Print and shaded views of the part. All mm, measured from the part's lowest x, y and z. Coordinates: 2 decimals unless noted, no trailing zeros. Write each loop counter-clockwise with the first axis right and the second up, starting at its lowest first coordinate (ties: lowest second). Pieces come first, ordered by that corner, then holes. Notation, with made-up numbers: (-17, 0) -> (6, 0) arc R24 ccw to (6, 36) -> close; hole circle Ø8 at (-4, 77). An arc over 180 degrees is marked (long way). Write item = value, one per line.
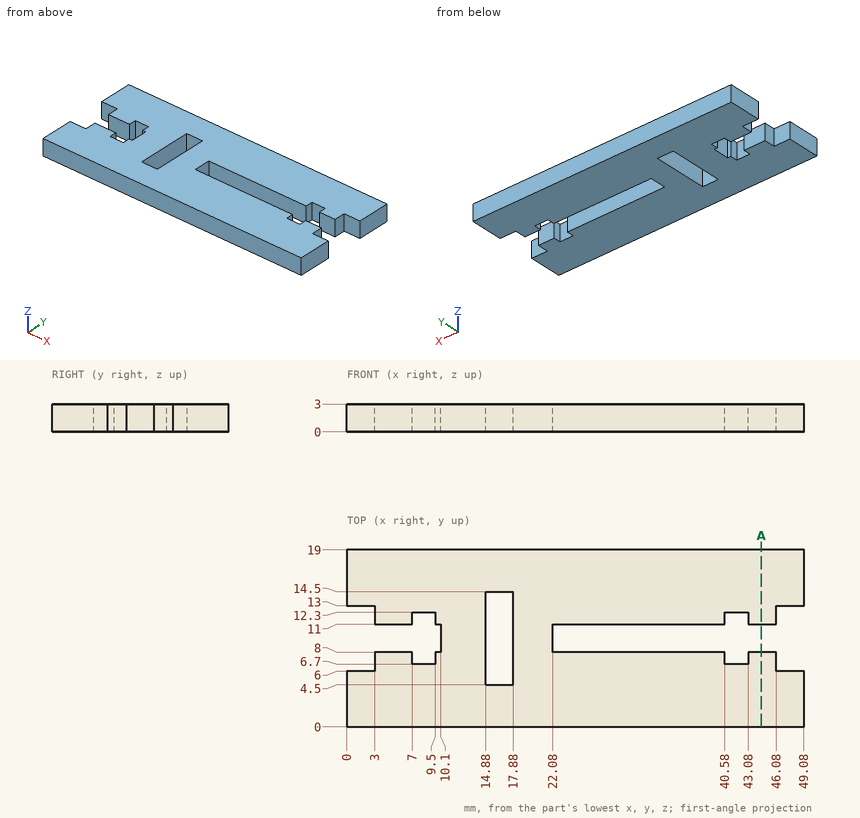
Q1. Pin check, flat tips, straight feed: pin 1 (0.6 mm diameter, centred on y = 11.5, z = 2, fed in from +X); pin 2 (0.6 mm diameter, centred on y = 12, z = 1, fed in from -X); pin 3 (0.9 mm diameter, centred on y = 10, z = 2, fed in from -X). Stop position of each tip, or through.
Model answer:
pin_1 = 46.08
pin_2 = 3
pin_3 = 10.1
Q2. Probe line 1 (X direction, y = 11.75, z = 2); line 2 (X direction, y = 14, z = 2.55); line 3 (Y direction, x = 29.5, z = 1.3). List the from-to ranges inside material, lowest first. Write a range as from..to.
Model answer:
line_1 = 3..7, 9.5..14.88, 17.88..40.58, 43.08..46.08
line_2 = 0..14.88, 17.88..49.08
line_3 = 0..8, 11..19
Q3. Saw through at A-A on x = 44.5. Give the cut face in (y, z), and give its area (3 significant figures).
Model answer:
outline = (0, 0) -> (8, 0) -> (8, 3) -> (0, 3) -> close; (11, 0) -> (19, 0) -> (19, 3) -> (11, 3) -> close
area = 48.0 mm²
